Autodesk Inventor part; units mm, degrees
ref_plane "YZ Plane" through (0, 0, 0) normal (1, 0, 0) x (0, 1, 0)
ref_plane "XZ Plane" through (0, 0, 0) normal (0, 1, 0) x (-1, 0, 0)
ref_plane "XY Plane" through (0, 0, 0) normal (0, 0, 1) x (1, 0, 0)
sketch "Base" plane through (0, 0, 0) normal (0, 0, 1) x (1, 0, 0)
  line L0 (-12.3981, -13.2027) -> (-12.3981, -7.9395)
  arc A0 (-12.3981, -13.2027) -> (15.9662, 8.5503) centre (0, 0) ccw
  arc A1 (15.9662, 8.5503) -> (5.3507, 16.1838) centre (0.6063, -1.6117) ccw
  arc A2 (5.3507, 16.1838) -> (-4.7343, 14.6301) centre (2.0791, 3.9125) ccw
  arc A3 (-4.7343, 14.6301) -> (-12.3981, -7.9395) centre (5.4695, -1.4207) ccw
  circle A4 centre (0, 0) radius 3
  circle A5 centre (0, 0) radius 3
  circle A6 centre (0, 0) radius 13.497 construction
  line L1 (-28.997, 27.4994) -> (26.303, 27.4994)
  line L2 (4.8764, -0.8461) -> (-14.6101, -0.8461)
  line L3 (-14.6101, -0.8461) -> (-28.997, 5.4994)
  line L4 (-28.997, 5.4994) -> (-28.997, 27.4994)
  line L5 (-28.997, 5.4994) -> (-11.7979, 11.6298)
  line L6 (-11.7979, 11.6298) -> (-2.5387, 11.6298)
  line L7 (-2.5387, 11.6298) -> (23.3778, 7.4994)
  line L8 (23.3778, 7.4994) -> (26.303, 7.4994)
  line L9 (26.303, 27.4994) -> (26.303, 7.4994)
  line L10 (4.8764, -0.8461) -> (26.303, 7.4994)
  line L11 (22.303, 23.4994) -> (9.7408, 23.4994)
  line L12 (9.7408, 23.4994) -> (13.5825, 13.7045)
  line L13 (13.5825, 13.7045) -> (19.1614, 13.7045)
  line L14 (19.1614, 13.7045) -> (22.303, 14.9367)
  line L15 (22.303, 14.9367) -> (22.303, 23.4994)
  line L16 (5.4441, 23.4994) -> (-1.5148, 23.4994)
  line L17 (-1.5148, 23.4994) -> (2.3269, 13.7045)
  line L18 (2.3269, 13.7045) -> (9.2858, 13.7045)
  line L19 (9.2858, 13.7045) -> (5.4441, 23.4994)
  circle A7 centre (-19.997, 19.4307) radius 2.5
  arc A8 (-4.7343, 14.6301) -> (-12.3981, -7.9395) centre (5.4695, -1.4207) ccw
  line L20 (-13.497, 0) -> (-13.497, -16.2978) construction
  point P0 (11.7017, -28.7626)
  point P1 (-13.5415, -0.8461)
  point P2 (15.8686, 8.6961)
  point P3 (-2.8782, -0.8461)
  point P4 (2.8782, -0.8461)
  point P5 (17.6358, 4.1236)
  dimension "d0" = 22
  dimension "d1" = 20
  dimension "d2" = 5
  dimension "d3" = 9
  dimension "d4" = 4
  dimension "d5" = 4
  dimension "d6" = 4
  dimension "d7" = 55.3
  dimension "d8" = 15.5
extrude "BaseFeature" add sketch "Base" along normal blind 18.2 contours L0 A3 L2 A4 L10 A0 | L10 L2 A4 A3 L6 L7 A1 A0 | L2 L3 L5 L6 A3 | L8 L7 A1 L19 L16 L17 A2 A3 L6 L5 L4 L1 L9 | A3 A2 L17 L18 L19 A1 L7 L6 | L19 L18 L17 A2 A1 | A1 A2 L17 L16 L19 | L15 L14 L13 L12 L11
extrude "ExtendFeature" add sketch "Base" along normal blind 23.72 contours L8 L7 A1 L19 L16 L17 A2 A3 L6 L5 L4 L1 L9 | A3 A2 L17 L18 L19 A1 L7 L6
extrude "Extend2Feature" add sketch "Base" against normal blind 5.2 contours L8 L7 A1 L19 L16 L17 A2 A3 L6 L5 L4 L1 L9 | A3 A2 L17 L18 L19 A1 L7 L6
sketch "PicatinnyRail" plane through (-28.997, 5.4994, 23.72) normal (-1, 0, 0) x (0, 0, 1)
  line L0 (-23.72, 0) -> (-5.52, 0)
  line L1 (-5.52, 0) -> (0, 0)
  line L2 (0, 22) -> (0, 0)
  line L3 (-28.92, 22) -> (0, 22) construction
  line L4 (-28.92, 0) -> (-28.92, 22)
  line L5 (-23.72, 0) -> (-28.92, 0)
  line L6 (-22.21, 14) -> (-6.71, 14)
  line L7 (-14.46, 14) -> (-14.46, 22) construction
  line L8 (-28.92, 22) -> (0, 22) construction
  line L9 (-28.92, 22) -> (0, 22) construction
  line L10 (-6.71, 14) -> (-3.71, 14) construction
  line L11 (0, 18) -> (0, 8.2052)
  line L12 (-22.21, 14) -> (-25.21, 14) construction
  line L13 (-3.71, 14) -> (-3.71, 17) construction
  line L14 (-25.21, 14) -> (-25.21, 17) construction
  line L15 (-23.72, 18) -> (-28.92, 18)
  line L16 (-6.71, 14) -> (-3.71, 17)
  line L17 (-22.21, 14) -> (-25.21, 17)
  line L18 (-3.71, 17) -> (-25.21, 17) construction
  line L19 (-3.71, 17) -> (-3.71, 18)
  line L20 (-25.21, 17) -> (-25.21, 18)
  line L21 (-3.71, 18) -> (-6.21, 20)
  line L22 (-3.71, 18) -> (-3.71, 20) construction
  line L23 (-3.71, 20) -> (-6.21, 20) construction
  line L24 (-6.21, 20) -> (-4.61, 22)
  line L25 (-25.21, 18) -> (-22.71, 20)
  line L26 (-22.71, 20) -> (-24.31, 22)
  line L27 (-24.31, 22) -> (-4.61, 22)
  point P0 (-23.72, -5.4994)
  dimension "d15" = 15.5
  dimension "d16" = 3
  dimension "d17" = 3
  dimension "d18" = 3
  dimension "d19" = 1
  dimension "d20" = 2
  dimension "d21" = 2.5
  dimension "d22" = 2
  dimension "d23" = 38.66
  dimension "d24" = 38.66
extrude "PicatinnyRailCut" cut sketch "PicatinnyRail" against normal through all
ref_plane "MidPlane" through (0, 0, 9.26) normal (0, 0, 1) x (1, 0, 0)
equation "\"d24\" = d23"
properties part number "SideHandleBase"
Check sheet for the modelled part. Datum: model origin and axes. Units: mm. A direction names the side the tool comes from. Give positions to 0.01 mm unless a question says otherwise; leave off trailing zeros. Write each loop counter-clockwise with the first axis right and the second up, starting at its lowest first coordinate (ties: lowest second). Pieces come first, ordered by that corner, then holes. Notation, with made-up numbers: (83.5, 66) -> (113.5, 66) arc R26 cw to (113.5, 81) -> close; hole circle Ø7 at (38.5, -30). An arc over 180 degrees is marked (long way). One line per item, written item: value. Start each with the question number.
Item 1: Section check C-C on x = -25.5. Record the cut outline in (y, z).
Item 2: Section check A-A on z = 11.5. Record the cut outline in (x, y), then the cut area to 3 significant figures.
Item 3: Material ranges on probe 1 along Y at (x, z) = (0, 11.25); probe 2 along Y at (x, z) = (-20, 21); probe 3 along Z at (x, y) = (15, -6), recorded low to high. Write a range as from..to.
Item 4: Section check D-D on y = 0. Record the cut outline in (x, z).
Item 5: Gauge pin test, flat ends, axial feed: pin 1 (6 mm diameter, centred on x = -22, z = 11, fed in from +Y); pin 2 (3.5 mm diameter, centred on x = 5.5, y = 17, fed in from +Z); pin 3 (5 mm diameter, centred on x = 0, y = 0, fed in from +Z); pin 4 (0.5 mm diameter, centred on x = -14, z = 12.5, fed in from -Y). Record the tip position at first contact, or that the pin passes through.
Item 6: Tool access check on faces 1 (the flat face through (-20.52, 8.52, -2.56)), 2 (the flat face through (16, 23.499, -3)), 3 (the flat face through (22.303, 19, 21)), 4 (the flat face through (-26, 19.499, 9)), 5 (the flat face through (-7, 11.63, 21)). Record the directions out of +Z, -Z, +X, -X, +Y, -Y that give a thin tool (end or side, any length) a straight path to the whole face; none if there is none.
Item 7: Section check B-B on y = 18. Record the cut outline in (x, z).
Item 8: Draft check along Y on faces 6 (the flat face through (-2, 19, 23.72)), 7 (the cylindrical face through (11.303, -14.152, 8.973)), 8 (the flat face through (25, 7.499, 9)). Enter one of: +Y half, -Y half, draft (parallel to the pull), parting line (faces both ways), or undercut.
Results list:
1. outline: (3.96, 0) -> (6.75, 0) -> (6.75, -5.2) -> (27.5, -5.2) -> (27.5, -0.59) -> (25.5, 1.01) -> (23.5, -1.49) -> (22.5, -1.49) -> (19.5, 1.51) -> (19.5, 17.01) -> (22.5, 20.01) -> (23.5, 20.01) -> (25.5, 17.51) -> (27.5, 19.11) -> (27.5, 23.72) -> (6.75, 23.72) -> (6.75, 18.2) -> (3.96, 18.2) -> close
2. outline: (-29, 5.5) -> (-14.61, -0.85) -> (-13.54, -0.85) arc R19.02 ccw to (-12.4, -7.94) -> (-12.4, -13.2) arc R18.11 ccw to (15.97, 8.55) arc R18.42 ccw to (15.87, 8.7) -> (23.38, 7.5) -> (26.3, 7.5) -> (26.3, 19.5) -> (-17.5, 19.5) arc R2.5 cw (long way) to (-22.5, 19.5) -> (-29, 19.5) -> close; hole circle Ø6 at (0, 0)
2. area: 1,410 mm²
3. probe 1: -18.11..-3, 3..19.5
3. probe 2: 8.71..16.93, 21.93..27.5
3. probe 3: 0..18.2
4. outline: (-16.53, 0) -> (-3, 0) -> (-3, 18.2) -> (-16.53, 18.2) -> close; (3, 0) -> (18.11, 0) -> (18.11, 18.2) -> (3, 18.2) -> close
5. pin 1: y = 19.5
5. pin 2: z = 18.2
5. pin 3: through
5. pin 4: y = -0.85
6. face 1: -Z, -Y
6. face 2: +Z, -Z
6. face 3: +Z
6. face 4: +X, -X, +Y
6. face 5: +Z, -Y
7. outline: (-29, -5.2) -> (-22.05, -5.2) -> (-22.05, 23.72) -> (-29, 23.72) -> close; (-17.95, -5.2) -> (0.64, -5.2) -> (0.64, 0) -> (7.6, 0) -> (7.6, -5.2) -> (11.9, -5.2) -> (11.9, 0) -> (22.3, 0) -> (22.3, -5.2) -> (26.3, -5.2) -> (26.3, 23.72) -> (22.3, 23.72) -> (22.3, 18.2) -> (11.9, 18.2) -> (11.9, 23.72) -> (7.6, 23.72) -> (7.6, 18.2) -> (0.64, 18.2) -> (0.64, 23.72) -> (-17.95, 23.72) -> close
8. face 6: draft
8. face 7: undercut
8. face 8: -Y half
